```python
from build123d import *

# Parameters (mm, degrees)
BOSS_EXTRUDE1_DEPTH = 108
LPATTERN1_COUNT     = 7
LPATTERN1_PITCH     = 15


with BuildPart() as part:
    # Sketch1 → Boss-Extrude1 (new body)
    with BuildSketch(Plane.XY):
        with BuildLine():
            Line((-3.5, 0), (3.5, 0))
            Line((3.5, 0), (3.5, 2.8))
            Line((3.5, 2.8), (3, 2.8))
            ThreePointArc((3, 2.8), (2.5, 3.3), (3, 3.8))
            Line((3, 3.8), (3.5, 3.8))
            Line((3.5, 3.8), (3.5, 4.8))
            Line((3.5, 4.8), (-3.5, 4.8))
            Line((-3.5, 4.8), (-3.5, 3.8))
            Line((-3.5, 3.8), (-3, 3.8))
            ThreePointArc((-3, 3.8), (-2.5, 3.3), (-3, 2.8))
            Line((-3, 2.8), (-3.5, 2.8))
            Line((-3.5, 2.8), (-3.5, 0))
        make_face()
    extrude(amount=-BOSS_EXTRUDE1_DEPTH)

    # Sketch2 → Cut-Revolve1 (revolve, cut)
    with BuildSketch(Plane(origin=(0, 0, 0), x_dir=(0, 0, -1), z_dir=(1, 0, 0))):
        Polygon((7.9, 4.8), (7.9, 2.5), (8.8, 2.5), (8.8, 0), (10, 0), (10, 4.8), align=None)
    cut_revolve1 = revolve(axis=Axis((0, 4.8, -10), (0, -1, 0)), mode=Mode.SUBTRACT)

    # LPattern1: Cut-Revolve1 ×7
    with Locations(*[(0, 0, -i * LPATTERN1_PITCH) for i in range(1, LPATTERN1_COUNT)]):
        add(cut_revolve1, mode=Mode.SUBTRACT)


solid = part.part
```
Could you check a few things on this model? Use its own coordinates, in mm. A direction names the side the tool comes from. Give positions to 0.01 mm unless a question says otherwise; leave off trailing zeros. Loops run counter-clockwise (first coordinate to the right, second up) from the corner with the lowest first, then second, coordinate; pieces in that order, holes last. Notation, with made-up numbers: (2.5, 36.25) - (27.5, 36.25) arc R8 cw to (27.5, 50.25) - close; hole circle Ø2 at (-6, 15). An arc over 180 degrees is marked (long way). Answer in a Markdown table with one row per item. Add a question column.
Q1. We'd pull the mould along Z, two halves only. Please class faces 1 (the face through (0, 2, 0)), 2 (the face through (-3.5, 1, -53)), 3 (the face through (-0.05, 1.23, -101.2)): +Z half, -Z half, draft (parallel to the pull), parting line (faces both ways), or undercut.
Q2. If we section it at A-A (z = -67): List the corners of the cut face in (x, y) for me, plus the area to 3 significant figures.
Q3. Which directions (+Z, -Z, +X, -X, +Y, -Y) give clear straight access to the entire face, cutting with the end or side of a thin tool? Please do faces 4 (the face through (-0.09, 3.63, -72.1)), 5 (the face through (0.46, 1.23, -68.89)).
Q4. For pin 1 (1 mm diameter, centred on y = 3.5, z = -63, fed in from -X), with a flat end and sliding along its axis, tell me the tip position at first contact or that it passes through.
Q5. Please list where these lines run through material, in increasing order: L1, parallel to X at y = 4, z = -25; L2, parallel to X at y = 3.4, z = -25; L3, parallel to Y at x = 3, z = -78. Write a range as from..to.
Q6. If we section it at C-C (x = 0): State how many separate pieces and enclosed holes the cut face has, plus the area to 3 significant figures.
Q7. If we section it at B-B (z = -40): List the corners of the cut face in (x, y) for me.
The answers:
| question | item | result |
|---|---|---|
| 1 | face 1 | +Z half |
| 1 | face 2 | draft |
| 1 | face 3 | undercut |
| 2 | outline | (-3.5, 0) - (3.5, 0) - (3.5, 2.8) - (3, 2.8) arc R0.5 cw to (3, 3.8) - (3.5, 3.8) - (3.5, 4.8) - (-3.5, 4.8) - (-3.5, 3.8) - (-3, 3.8) arc R0.5 cw to (-3, 2.8) - (-3.5, 2.8) - close |
| 2 | area | 31.8 mm^2 |
| 3 | face 4 | +Y |
| 3 | face 5 | +Y, -Y |
| 4 | pin 1 | stops at x = -3.5 |
| 5 | L1 | x = -3.5..-2.1, 2.1..3.5 |
| 5 | L2 | x = -2.51..-2.1, 2.1..2.51 |
| 5 | L3 | y = 0..2.8, 3.8..4.8 |
| 6 | separate pieces | 8 |
| 6 | enclosed holes | 0 |
| 6 | area | 409 mm^2 |
| 7 | outline | (-3.5, 0) - (-1.2, 0) - (-1.2, 2.5) - (-2.1, 2.5) - (-2.1, 4.8) - (-3.5, 4.8) - (-3.5, 3.8) - (-3, 3.8) arc R0.5 cw to (-3, 2.8) - (-3.5, 2.8) - close; (1.2, 0) - (3.5, 0) - (3.5, 2.8) - (3, 2.8) arc R0.5 cw to (3, 3.8) - (3.5, 3.8) - (3.5, 4.8) - (2.1, 4.8) - (2.1, 2.5) - (1.2, 2.5) - close |
